from build123d import *

# Parameters (mm, degrees)
SKETCH_1_W          = 57.3
SKETCH_1_H          = 61.6
EXTRUDE_1_DEPTH     = 2.8
SKETCH_1_11_W       = 57.3
SKETCH_1_11_H       = 61.6
SKETCH_1_11_W_2     = 53.9
SKETCH_1_11_H_2     = 58.2
EXTRUDE_1_2_DEPTH   = 14.9
SKETCH_1_13_W       = 3
SKETCH_1_13_H       = 6.8
CUT_EXTRUDE_1_DEPTH = 2.8
SKETCH_1_14_W       = 1.4
SKETCH_1_14_H       = 61.6
EXTRUDE_2_DEPTH     = 10
SKETCH_1_15_R       = 1.9
CUT_EXTRUDE_2_DEPTH = 45.625917358
CHAMFER_1_SIZE      = 1


with BuildPart() as part:
    # 草图1 → Extrude 1 (new body)
    with BuildSketch(Plane(origin=(0, 0, 0), x_dir=(1, 0, 0), z_dir=(0, 1, 0))):
        Rectangle(SKETCH_1_W, SKETCH_1_H)
    extrude(amount=EXTRUDE_1_DEPTH)

    # 草图1<11> → Extrude 1 2 (add)
    with BuildSketch(Plane(origin=(0, 0, 0), x_dir=(1, 0, 0), z_dir=(0, 1, 0))):
        Rectangle(SKETCH_1_11_W, SKETCH_1_11_H)
        Rectangle(SKETCH_1_11_W_2, SKETCH_1_11_H_2, mode=Mode.SUBTRACT)
    extrude(amount=EXTRUDE_1_2_DEPTH)

    # 草图1<13> → 切除-拉伸1 (cut)
    with BuildSketch(Plane(origin=(0, 0, 0), x_dir=(1, 0, 0), z_dir=(0, 1, 0))):
        with Locations((-16.025, -27.4)):
            Rectangle(SKETCH_1_13_W, SKETCH_1_13_H)
        with Locations((-11.625, -27.4)):
            Rectangle(SKETCH_1_13_W, SKETCH_1_13_H)
    extrude(amount=CUT_EXTRUDE_1_DEPTH, mode=Mode.SUBTRACT)

    # 草图1<14> → 凸台-拉伸2 (add)
    with BuildSketch(Plane(origin=(0, 0, 0), x_dir=(1, 0, 0), z_dir=(0, 1, 0))):
        with Locations((-13.825, 0)):
            Rectangle(SKETCH_1_14_W, SKETCH_1_14_H)
        with Locations((13.825, 0)):
            Rectangle(SKETCH_1_14_W, SKETCH_1_14_H)
        Rectangle(SKETCH_1_14_W, SKETCH_1_14_H)
    extrude(amount=EXTRUDE_2_DEPTH)

    # 草图1<15> → 切除-拉伸2 (cut, through all)
    with BuildSketch(Plane(origin=(0, 0, 0), x_dir=(1, 0, 0), z_dir=(0, 1, 0))):
        with Locations(Location((-20.7375, 0, 0), (0, 0, 270))):
            Circle(SKETCH_1_15_R)
        with Locations(Location((-6.9125, 0, 0), (0, 0, 270))):
            Circle(SKETCH_1_15_R)
        with Locations(Location((6.9125, 0, 0), (0, 0, 270))):
            Circle(SKETCH_1_15_R)
        with Locations(Location((20.7375, 0, 0), (0, 0, 270))):
            Circle(SKETCH_1_15_R)
    extrude(amount=CUT_EXTRUDE_2_DEPTH, mode=Mode.SUBTRACT)

    # 倒角1
    chamfer_1_edges = [part.edges().sort_by_distance(p)[0] for p in [
        (-20.7375, 2.8, -1.9),
        (-6.9125, 2.8, -1.9),
        (6.9125, 2.8, -1.9),
        (20.7375, 2.8, -1.9),
    ]]
    chamfer(chamfer_1_edges, length=CHAMFER_1_SIZE)


solid = part.part
Source: CAD feature listing. Evaluate the final solid. Frame: model axes, mm. A direction names the side the tool comes from. Coordinates: 2 decimals unless noted, no trailing zeros. Order: outer loops, then holes, each group sorted by start corner. A loop starts at its lowest first (then second) coordinate and runs counter-clockwise, first axis right, second up. Notation, with made-up numbers: M 54,22.5 L 58,22.5 A27 cw 58,59.5 Z; hole C -22.5,-28.5 d11. An arc over 180 degrees is marked long. Write each question's results on one line, items separated by ' | '. Start each with the question number.
Item 1: Cut plane D-D (y = 12). Return loops of the section in (x, z).
Item 2: Cut plane C-C (z = 0). Count the separate pieces of the cut face and the enclosed holes in it, and give its area (3 significant figures).
Item 3: Line query: probe 1 along X at (y, z) = (9.75, -13) (3 decimals); probe 2 along X at (y, z) = (0.95, 0); probe 3 along X at (y, z) = (2.25, 27) (3 decimals). Output: solid intervals per line, ascending.
Item 4: Cut plane A-A (y = 9). Return loops of the section in (x, z) (3 decimals).
Item 5: Cut plane B-B (x = -12). Return loops of the section in (y, z), and give its area (3 significant figures).
Item 6: Draft query along X for faces 5 (the face through (3, 2.8, 0)), 6 (the face through (-28, 14.9, 0)). Return one class per face: pulls with the +X half, pulls with the -X half, needs draft (parallel to the pull), parting line crosses it, or undercut.
Item 7: Set-up query: faces 1 (the face through (5.058, 0.887, -0.412)), 2 (the face through (-12, 1, 24)), 3 (the face through (-25, 2.8, 0)), 4 (the face through (-16, 2.8, 30)). Return all of +Z, -Z, +X, -X, +Y, -Y with unobstructed straight access to the full face (end or side cutting, diameter ignored); none if empty.
Item 8: First-contact query: pin 1 Ø1.4 at (x, z) = (-11, 30) entering from -Y; pin 2 Ø10 at (x, z) = (-19, -2.5) entering from +Y; pin 3 Ø3.5 at (x, z) = (20, -7.5) entering from +Y. Flat tips, straight axial feed; report the tip coordinate or a pass-through.
Checked values:
1) outline: M -28.65,-30.8 L 28.65,-30.8 L 28.65,30.8 L -28.65,30.8 Z; hole M -26.95,-29.1 L 26.95,-29.1 L 26.95,29.1 L -26.95,29.1 Z
2) separate pieces: 5 | enclosed holes: 0 | area: 185 mm2
3) probe 1: x = -28.65 to -26.95, -14.525 to -13.125, -0.7 to 0.7, 13.125 to 14.525, 26.95 to 28.65 | probe 2: x = -28.65 to -22.64, -18.84 to -8.81, -5.01 to 5.01, 8.81 to 18.84, 22.64 to 28.65 | probe 3: x = -28.65 to -17.525, -14.525 to -13.125, -10.125 to 28.65
4) outline: M -28.65,-30.8 L 28.65,-30.8 L 28.65,30.8 L -28.65,30.8 Z; hole M -26.95,-29.1 L -14.525,-29.1 L -14.525,29.1 L -26.95,29.1 Z; hole M -13.125,-29.1 L -0.7,-29.1 L -0.7,29.1 L -13.125,29.1 Z; hole M 0.7,-29.1 L 13.125,-29.1 L 13.125,29.1 L 0.7,29.1 Z; hole M 14.525,-29.1 L 26.95,-29.1 L 26.95,29.1 L 14.525,29.1 Z
5) outline: M 0,-30.8 L 14.9,-30.8 L 14.9,-29.1 L 2.8,-29.1 L 2.8,24 L 0,24 Z; M 2.8,29.1 L 14.9,29.1 L 14.9,30.8 L 2.8,30.8 Z | area: 195 mm2
6) face 5: undercut | face 6: needs draft
7) face 1: +Y, -Y | face 2: +Z, +Y, -Y | face 3: +Y | face 4: +Z, -Y
8) pin 1: stops at y = 2.8 | pin 2: stops at y = 10 | pin 3: stops at y = 2.8
